Part model, mm, in its own coordinate system. A direction names the side the tool comes from. Coordinates: 2 decimals unless noted, no trailing zeros. Loops run counter-clockwise (first coordinate to the right, second up) from the corner with the lowest first, then second, coordinate; pieces in that order, holes last. Notation, with made-up numbers: M 78.25,38 L 110.25,38 A21 cw 110.25,48 Z; hole C 25,8 d2. An arc over 180 degrees is marked long. Answer as a JSON object with one key per item and string values. Group by question number.
1. Mould opens along Y. For faces 6 (the face through (6, 9, 15)), 7 (the face through (3.45, -38.05, 0.21)), 8 (the face through (6.844, 7.227, -7.418)), 9 (the face through (5.79, 18.55, -6.54)) say: released by +Y, released by -Y, zero draft, split by the parting line, or undercut.
2. Saw through at A-A on x = -3.5. Write the cut outline in (y, z), then the cut area to 3 significant figures.
3. Drill centre lines: L1, parallel to Z at x = 6.25, y = 7.5; L2, parallel to Y at x = 2.75, z = -1; L3, parallel to Y at x = 10.75, z = -4.5. Where is each one in solid material? Low to high.
4. 3-axis set-ups, long thin cutter, end or side, ignore diameter. For faces 1 (the face through (1, 36.37, 6.54)), 2 (the face through (4.5, -24.9, 13.6)), 3 (the face through (10.5, -25, -7)), 4 (the face through (7.5, 25.16, 0.17)), 5 (the face through (0, 34, 6)): which of +Z, -Z, +X, -X, +Y, -Y reach the whole face in a straight line?
5. Saw through at C-C on y = 25. Write the cut outline in (x, z).
6. Drop flat-ended pins along their axis: pin 1 Ø2.5 at (y, z) = (-25, -7.5) entering from +X; pin 2 Ø1 at (y, z) = (-30.5, -11.5) entering from -X; pin 3 Ø1.4 at (y, z) = (31.5, 14) entering from -X; pin 4 Ø4 at (y, z) = (7.5, 9.5) entering from +X. Give the stop position or say it passes through.
7. Saw through at B-B on y = 7.5. Write the cut outline in (x, z).
8. Saw through at D-D on z = -3. Write the cut outline in (x, y), then the cut area to 3 significant figures.
from build123d import *

# Parameters (mm, degrees)
BOSS_EXTRUDE1_DEPTH     = 15
BOSS_EXTRUDE2_DEPTH     = 2.75
CUT_EXTRUDE1_START      = -6
CUT_EXTRUDE1_DEPTH      = 5
SKETCH5_W               = 5
SKETCH5_H               = 8.618802154
CUT_EXTRUDE2_DEPTH      = 3
MIRROR5_START           = -6
MIRROR5_COPY_1_DEPTH    = 5
MIRROR5_COPY_2_SKETCH_W = 5
MIRROR5_COPY_2_SKETCH_H = 8.618802154
MIRROR5_COPY_2_DEPTH    = 3
SKETCH6_R               = 2.1
CUT_EXTRUDE3_DEPTH      = 44.468379312
LPATTERN2_COUNT         = 2
LPATTERN2_PITCH         = 16
BOSS_EXTRUDE3_DEPTH     = 30
SKETCH9_W               = 8
SKETCH9_H               = 6
SKETCH9_W_2             = 6
BOSS_EXTRUDE4_DEPTH     = 14
SKETCH10_W              = 30
SKETCH10_H              = 6
BOSS_EXTRUDE5_DEPTH     = 6
CHAMFER1_SIZE           = 2.5
CHAMFER2_SIZE           = 7
CHAMFER2_SIZE2          = 5.873697418


with BuildPart() as part:
    # Sketch1 → Boss-Extrude1 (new, symmetric)
    with BuildSketch(Plane.XY):
        with BuildLine():
            Line((13.5, -25), (13.5, 25))
            Line((13.5, 25), (13.5, 32.794228634))
            Line((13.5, 32.794228634), (6.75, 36.691342951))
            ThreePointArc((6.75, 36.691342951), (3.494057109, 38.039998655), (0, 38.5))
            Line((0, 38.5), (0, 32.5))
            ThreePointArc((0, 32.5), (7.5, 25), (0, 17.5))
            Line((0, 17.5), (0, -17.5))
            ThreePointArc((0, -17.5), (7.5, -25), (0, -32.5))
            Line((0, -32.5), (0, -38.5))
            ThreePointArc((0, -38.5), (3.494057109, -38.039998655), (6.75, -36.691342951))
            Line((6.75, -36.691342951), (13.5, -32.794228634))
            Line((13.5, -32.794228634), (13.5, -25))
        make_face()
    extrude(amount=BOSS_EXTRUDE1_DEPTH, both=True)

    # Sketch2 → Boss-Extrude2 (add)
    with BuildSketch(Plane.XY.offset(15)):
        with BuildLine():
            Line((0, 32.5), (0, 29.5))
            ThreePointArc((0, 29.5), (4.5, 25), (0, 20.5))
            Line((0, 20.5), (0, 17.5))
            ThreePointArc((0, 17.5), (7.5, 25), (0, 32.5))
        make_face()
        with BuildLine():
            Line((0, -17.5), (0, -20.5))
            ThreePointArc((0, -20.5), (4.5, -25), (0, -29.5))
            Line((0, -29.5), (0, -32.5))
            ThreePointArc((0, -32.5), (7.5, -25), (0, -17.5))
        make_face()
    boss_extrude2 = extrude(amount=-BOSS_EXTRUDE2_DEPTH)

    # Mirror1: Boss-Extrude2 across plane
    add(boss_extrude2.mirror(Plane.XY))

    # Sketch3 → Cut-Extrude1 (cut)
    with BuildSketch(Plane.XY.offset(15).offset(CUT_EXTRUDE1_START)):
        with BuildLine():
            Line((0, 34.5), (0, 36.5))
            ThreePointArc((0, 36.5), (1.009892189, 36.367045171), (1.950961894, 35.977241336))
            Line((1.950961894, 35.977241336), (13.5, 29.309401077))
            Line((13.5, 29.309401077), (13.5, 27))
            Line((13.5, 27), (0.950961894, 34.245190528))
            ThreePointArc((0.950961894, 34.245190528), (0.492254099, 34.435193518), (0, 34.5))
        make_face()
        with BuildLine():
            Line((13.5, 23), (0.950961894, 15.754809472))
            ThreePointArc((0.950961894, 15.754809472), (0.492254099, 15.564806482), (0, 15.5))
            Line((0, 15.5), (0, 13.5))
            ThreePointArc((0, 13.5), (1.009892189, 13.632954829), (1.950961894, 14.022758664))
            Line((1.950961894, 14.022758664), (13.5, 20.690598923))
            Line((13.5, 20.690598923), (13.5, 23))
        make_face()
    cut_extrude1 = extrude(amount=-CUT_EXTRUDE1_DEPTH, mode=Mode.SUBTRACT)

    # Sketch5 → Cut-Extrude2 (cut)
    with BuildSketch(Plane(origin=(13.5, 0, 0), x_dir=(0, 0, -1), z_dir=(1, 0, 0))):
        with Locations((-6.5, 25)):
            Rectangle(SKETCH5_W, SKETCH5_H)
    cut_extrude2 = extrude(amount=-CUT_EXTRUDE2_DEPTH, mode=Mode.SUBTRACT)

    # Mirror3: Cut-Extrude1, Cut-Extrude2 across plane
    add(cut_extrude1.mirror(Plane.XY), mode=Mode.SUBTRACT)
    add(cut_extrude2.mirror(Plane.XY), mode=Mode.SUBTRACT)

    # Mirror5: Cut-Extrude1, Cut-Extrude2 across plane
    add(cut_extrude1.mirror(Plane.ZX), mode=Mode.SUBTRACT)
    add(cut_extrude2.mirror(Plane.ZX), mode=Mode.SUBTRACT)

    # Mirror5 copy 1 sketch → Mirror5 copy 1 (cut)
    with BuildSketch(Plane(origin=(0, 0, -15), x_dir=(1, 0, 0), z_dir=(0, 0, -1)).offset(MIRROR5_START)):
        with BuildLine():
            Line((0, 34.5), (0, 36.5))
            ThreePointArc((0, 36.5), (1.009892189, 36.367045171), (1.950961894, 35.977241336))
            Line((1.950961894, 35.977241336), (13.5, 29.309401077))
            Line((13.5, 29.309401077), (13.5, 27))
            Line((13.5, 27), (0.950961894, 34.245190528))
            ThreePointArc((0.950961894, 34.245190528), (0.492254099, 34.435193518), (0, 34.5))
        make_face()
        with BuildLine():
            Line((13.5, 23), (0.950961894, 15.754809472))
            ThreePointArc((0.950961894, 15.754809472), (0.492254099, 15.564806482), (0, 15.5))
            Line((0, 15.5), (0, 13.5))
            ThreePointArc((0, 13.5), (1.009892189, 13.632954829), (1.950961894, 14.022758664))
            Line((1.950961894, 14.022758664), (13.5, 20.690598923))
            Line((13.5, 20.690598923), (13.5, 23))
        make_face()
    extrude(amount=-MIRROR5_COPY_1_DEPTH, mode=Mode.SUBTRACT)

    # Mirror5 copy 2 sketch → Mirror5 copy 2 (cut)
    with BuildSketch(Plane(origin=(13.5, 0, 0), x_dir=(0, 0, 1), z_dir=(1, 0, 0))):
        with Locations((-6.5, 25)):
            Rectangle(MIRROR5_COPY_2_SKETCH_W, MIRROR5_COPY_2_SKETCH_H)
    extrude(amount=-MIRROR5_COPY_2_DEPTH, mode=Mode.SUBTRACT)

    # Sketch6 → Cut-Extrude3 (cut, through all)
    with BuildSketch(Plane(origin=(13.5, 0, 0), x_dir=(0, 0, -1), z_dir=(1, 0, 0))):
        with Locations(Location((-9.5, -8.5, 0), (0, 0, 90))):
            Circle(SKETCH6_R)
        with Locations(Location((9.5, -8.5, 0), (0, 0, 90))):
            Circle(SKETCH6_R)
    cut_extrude3 = extrude(amount=-CUT_EXTRUDE3_DEPTH, mode=Mode.SUBTRACT)

    # LPattern2: Cut-Extrude3 ×2
    with Locations(*[(0, i * LPATTERN2_PITCH, 0) for i in range(1, LPATTERN2_COUNT)]):
        add(cut_extrude3, mode=Mode.SUBTRACT)

    # Sketch8 → Boss-Extrude3 (add)
    with BuildSketch(Plane.XY.offset(15)):
        with BuildLine():
            Line((0, 38.5), (13.5, 38.5))
            Line((13.5, 38.5), (13.5, 32.794228634))
            Line((13.5, 32.794228634), (6.75, 36.691342951))
            ThreePointArc((6.75, 36.691342951), (3.494057109, 38.039998655), (0, 38.5))
        make_face()
    extrude(amount=-BOSS_EXTRUDE3_DEPTH)

    # Sketch9 → Boss-Extrude4 (add)
    with BuildSketch(Plane.ZY):
        with Locations((0, 35.5)):
            Rectangle(SKETCH9_W, SKETCH9_H)
        with Locations((12, 35.5)):
            Rectangle(SKETCH9_W_2, SKETCH9_H)
        with Locations((-12, 35.5)):
            Rectangle(SKETCH9_W_2, SKETCH9_H)
    extrude(amount=BOSS_EXTRUDE4_DEPTH)

    # Sketch10 → Boss-Extrude5 (add)
    with BuildSketch(Plane.ZY.offset(14)):
        with Locations((0, 35.5)):
            Rectangle(SKETCH10_W, SKETCH10_H)
    extrude(amount=-BOSS_EXTRUDE5_DEPTH)

    # Chamfer1
    chamfer1_edges = [part.edges().sort_by_distance(p)[0] for p in [
        (-8, 35.5, 4),
        (-8, 35.5, 9),
        (-8, 35.5, -4),
        (-8, 35.5, -9),
    ]]
    chamfer(chamfer1_edges, length=CHAMFER1_SIZE - 0.0001)  # a hair under: the kernel refuses the full size

    # Chamfer2
    chamfer2_edges = [part.edges().sort_by_distance(p)[0] for p in [
        (13.5, 38.5, 0),
    ]]
    chamfer2_side = [part.faces().sort_by_distance(p)[0] for p in [
        (0.031912143, 38.5, 0),
    ]]
    chamfer(chamfer2_edges, length=CHAMFER2_SIZE, length2=CHAMFER2_SIZE2, reference=chamfer2_side[0])


solid = part.part
Outcome:
{
 "1": {"face 6": "zero draft", "face 7": "released by -Y", "face 8": "undercut", "face 9": "undercut"},
 "2": {"outline": "M 32.5,-15 L 38.5,-15 L 38.5,-9 L 32.5,-9 Z; M 32.5,-4 L 38.5,-4 L 38.5,4 L 32.5,4 Z; M 32.5,9 L 38.5,9 L 38.5,15 L 32.5,15 Z", "area": "120 mm²"},
 "3": {"L1": "z = -15 to -11.6, -7.4 to 7.4, 11.6 to 15", "L2": "y = -38.22 to -31.98, -18.02 to 18.02, 31.98 to 38.5", "L3": "y = -34.38 to -30.9, -19.1 to 19.1, 30.9 to 34.93"},
 "4": {"face 1": "none", "face 2": "+Z, -Z, -X", "face 3": "+X", "face 4": "-X", "face 5": "+Y, -Y"},
 "5": {"outline": "M 4.5,-15 L 13.5,-15 L 13.5,-9 L 10.5,-9 L 10.5,-4 L 13.5,-4 L 13.5,4 L 10.5,4 L 10.5,9 L 13.5,9 L 13.5,15 L 4.5,15 L 4.5,12.25 L 7.5,12.25 L 7.5,-12.25 L 4.5,-12.25 Z"},
 "6": {"pin 1": "stops at x = 10.5", "pin 2": "stops at x = 4.5", "pin 3": "stops at x = 0", "pin 4": "passes through"},
 "7": {"outline": "M 0,-15 L 13.5,-15 L 13.5,-11.6 L 0,-11.6 Z; M 0,-7.4 L 13.5,-7.4 L 13.5,7.4 L 0,7.4 Z; M 0,11.6 L 13.5,11.6 L 13.5,15 L 0,15 Z"},
 "8": {"outline": "M -14,32.5 L 0,32.5 A7.5 cw 0,17.5 L 0,-17.5 A7.5 cw 0,-32.5 L 0,-38.5 A13.5 ccw 6.75,-36.69 L 13.5,-32.79 L 13.5,32.63 L 6.5,38.5 L -14,38.5 Z", "area": "897 mm²"}
}
